Here's how the part is built. I have some questions about the finished solid (model axes, mm). Face numbers are marked on the shaded views. A direction names the side the tool comes from. Round coordinates to 2 decimals unless told otherwise and drop trailing zeros. Order: outer loops, then holes, each group sorted by start corner. A loop starts at its lowest first (then second) coordinate and runs counter-clockwise, first axis right, second up. Notation, with made-up numbers: (24, 42) -> (72, 42) arc R28 cw to (72, 77) -> close; hole circle Ø4 at (-17, 11.5). An arc over 180 degrees is marked (long way). One line per item, written item: value.
```python
from build123d import *

# Parameters (mm, degrees)
SKETCH_1_W          = 12
SKETCH_1_H          = 10
EXTRUDE_1_DEPTH     = 15
FILLET_1_R          = 1
SKETCH_2_R          = 1.3
SKETCH_2_R_2        = 0.8
EXTRUDE_2_DEPTH     = 8
EXTRUDE_3_DEPTH     = 1.2
SKETCH_6_R          = 0.8
CUT_EXTRUDE_1_DEPTH = 1.2
SKETCH_7_R          = 1.5
EXTRUDE_4_DEPTH     = 55


with BuildPart() as part:
    # 草图1 → 凸台-拉伸1 (new body)
    with BuildSketch(Plane.XY):
        with Locations((6, 5)):
            Rectangle(SKETCH_1_W, SKETCH_1_H)
    extrude(amount=EXTRUDE_1_DEPTH)

    # 圆角1
    fillet_1_edges = [part.edges().sort_by_distance(p)[0] for p in [
        (12, 5, 15),
        (6, 10, 15),
        (0, 5, 15),
        (6, 10, 0),
        (12, 5, 0),
        (6, 0, 0),
        (0, 5, 0),
        (6, 0, 15),
        (0, 10, 7.5),
        (12, 10, 7.5),
        (12, 0, 7.5),
        (0, 0, 7.5),
    ]]
    fillet(fillet_1_edges, radius=FILLET_1_R)

    # 草图2 → 凸台-拉伸2 (add)
    with BuildSketch(Plane(origin=(0, 0, 0), x_dir=(-1, 0, 0), z_dir=(0, 0, -1))):
        with Locations((-2.927114882, 2.439262401)):
            Circle(SKETCH_2_R)
        with Locations((-2.927114882, 2.439262401)):
            Circle(SKETCH_2_R_2, mode=Mode.SUBTRACT)
        with Locations((-9.072885118, 7.560737599)):
            Circle(SKETCH_2_R)
        with Locations((-9.072885118, 7.560737599)):
            Circle(SKETCH_2_R_2, mode=Mode.SUBTRACT)
    extrude(amount=EXTRUDE_2_DEPTH)

    # 草图3 → 凸台-拉伸3 (add)
    with BuildSketch(Plane(origin=(0, 0, -8), x_dir=(-1, 0, 0), z_dir=(0, 0, -1))):
        Polygon((0, 0.5), (-0.5, 0), (-11.5, 0), (-12, 0.5), (-12, 9.5), (-11.5, 10), (-0.5, 10), (0, 9.5), align=None)
    extrude(amount=EXTRUDE_3_DEPTH)

    # 草图6 → 切除-拉伸1 (cut)
    with BuildSketch(Plane(origin=(0, 0, -9.2), x_dir=(-1, 0, 0), z_dir=(0, 0, -1))):
        with Locations((-2.927114882, 2.439262401)):
            Circle(SKETCH_6_R)
        with Locations((-9.072885118, 7.560737599)):
            Circle(SKETCH_6_R)
    extrude(amount=-CUT_EXTRUDE_1_DEPTH, mode=Mode.SUBTRACT)

    # 草图7 → 凸台-拉伸4 (add)
    with BuildSketch(Plane.XY.offset(-9.2)):
        with Locations((6, 5)):
            Circle(SKETCH_7_R)
    extrude(amount=-EXTRUDE_4_DEPTH)


solid = part.part
```
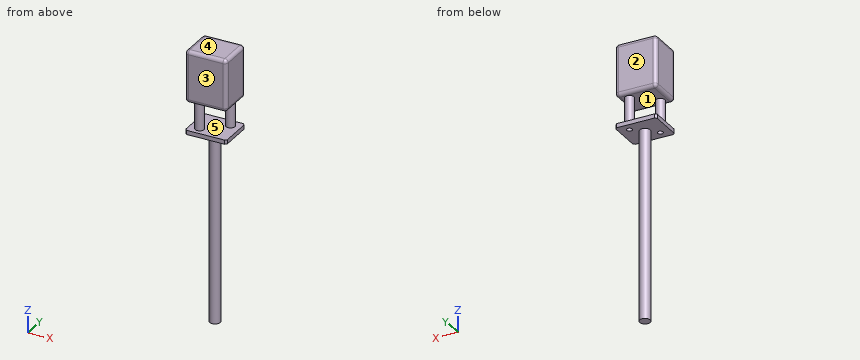
Q1. Which directions (+Z, -Z, +X, -X, +Y, -Y) give clear straight access to the entire face, cutting with the end or side of a thin tool? Please do the marked faces 4 and 5.
Answers:
face 4: +Z, +X, -X, +Y, -Y
face 5: none
Q2. I want a section at B-B on y = 5. Write out the boundary of the cut face in (x, z).
Answers:
outline: (0, -9.2) -> (4.5, -9.2) -> (4.5, -64.2) -> (7.5, -64.2) -> (7.5, -9.2) -> (12, -9.2) -> (12, -8) -> (0, -8) -> close; (0, 1) arc R1 ccw to (1, 0) -> (11, 0) arc R1 ccw to (12, 1) -> (12, 14) arc R1 ccw to (11, 15) -> (1, 15) arc R1 ccw to (0, 14) -> close
Q3. I want a section at C-C on z = -3.5. Write out the boundary of the cut face in (x, y).
Answers:
outline: circle Ø2.6 at (2.93, 2.44); circle Ø2.6 at (9.07, 7.56); hole circle Ø1.6 at (2.93, 2.44); hole circle Ø1.6 at (9.07, 7.56)
Q4. I need wall thicknesses on line 1 along Z through (x, y) = (5.25, 8.25); line 2 along Z through (x, y) = (5.5, 4); line 3 along X through (y, z) = (7, -8.5). Which ranges of each line are inside material? Lowest first, please.
Answers:
line 1: -9.2 to -8, 0 to 15
line 2: -64.2 to -8, 0 to 15
line 3: 0 to 8.5, 9.64 to 12
Q5. If we mould it in two halves opening along Y, with no side actions, what happens to the marked faces 1, 2 and 3? For each: pulls with the +Y half, pulls with the -Y half, needs draft (parallel to the pull), parting line crosses it, or undercut.
Answers:
face 1: needs draft
face 2: pulls with the +Y half
face 3: pulls with the -Y half
Q6. I want a section at D-D on z = -28.5. Write out the boundary of the cut face in (x, y).
Answers:
outline: circle Ø3 at (6, 5)
Q7. I want a section at A-A on x = 6. Write out the boundary of the cut face in (y, z).
Answers:
outline: (0, -9.2) -> (3.5, -9.2) -> (3.5, -64.2) -> (6.5, -64.2) -> (6.5, -9.2) -> (10, -9.2) -> (10, -8) -> (0, -8) -> close; (0, 1) arc R1 ccw to (1, 0) -> (9, 0) arc R1 ccw to (10, 1) -> (10, 14) arc R1 ccw to (9, 15) -> (1, 15) arc R1 ccw to (0, 14) -> close
Q8. For P1, Ø3, axis at x = 3.5, z = -40.5, coming from the +Y side; P2, Ø1.8, axis at x = 9.07, y = 7.56, coming from the -Z side; P3, Ø2.5, axis at x = 7.5, y = 3.5, coming from the -Z side; P4, Ø1.3, axis at x = 3, y = 2.5, coming from the -Z side, each with a flat end and sliding along its axis, tell me the tip position at first contact or that it passes through.
Answers:
P1: y = 6.12
P2: z = -9.2
P3: z = -64.2
P4: z = 0
